Here's how the part is built. I have some questions about the finished solid (model axes, mm). A direction names the side the tool comes from. Coordinates: 2 decimals unless noted, no trailing zeros. Loops run counter-clockwise (first coordinate to the right, second up) from the corner with the lowest first, then second, coordinate; pieces in that order, holes last. Notation, with made-up numbers: (82.5, 0) - (120.5, 0) arc R24 cw to (120.5, 35) - close; hole circle Ø7 at (47, 30). An arc over 180 degrees is marked (long way). Use a Markdown table: item, result.
```python
from build123d import *

# Parameters (mm, degrees)
SKETCH2_R           = 3.429
BOSS_EXTRUDE1_DEPTH = 6.35
SKETCH6_R           = 3.429
BOSS_EXTRUDE2_DEPTH = 6.35
SKETCH7_R           = 2.63525
BOSS_EXTRUDE3_DEPTH = 11.43
CUT_EXTRUDE2_START  = -6.35
CUT_EXTRUDE2_DEPTH  = 6.35
FILLET2_R           = 2.54
FILLET3_R           = 0.508
SKETCH12_R          = 3.302
CUT_EXTRUDE3_DEPTH  = 15.875
SKETCH13_R          = 3.302
CUT_EXTRUDE4_DEPTH  = 15.875


with BuildPart() as part:
    # Sketch2 → Boss-Extrude1 (new body)
    with BuildSketch(Plane(origin=(0, 0, 0), x_dir=(1, 0, 0), z_dir=(0, 1, 0))):
        with BuildLine():
            Line((-7.239, 0), (-7.239, 10.16))
            ThreePointArc((-7.239, 10.16), (0, 17.399), (7.239, 10.16))
            Line((7.239, 10.16), (7.239, 0))
            Line((7.239, 0), (-7.239, 0))
        make_face()
        with Locations(Location((0, 10.16, 0), (0, 0, 270))):
            Circle(SKETCH2_R, mode=Mode.SUBTRACT)
    extrude(amount=BOSS_EXTRUDE1_DEPTH)



with BuildPart() as body_2:
    # Sketch6 → Boss-Extrude2 (new body)
    with BuildSketch(Plane(origin=(0, 31.242, 0), x_dir=(-1, 0, 0), z_dir=(0, -1, 0))):
        with BuildLine():
            Line((7.239, 0), (-7.239, 0))
            Line((-7.239, 0), (-7.239, 10.16))
            ThreePointArc((-7.239, 10.16), (0, 17.399), (7.239, 10.16))
            Line((7.239, 10.16), (7.239, 0))
        make_face()
        with Locations(Location((0, 10.16, 0), (0, 0, 270))):
            Circle(SKETCH6_R, mode=Mode.SUBTRACT)
    extrude(amount=BOSS_EXTRUDE2_DEPTH)


with BuildPart() as part_1:
    add(part.part)

    add(body_2.part)  # Boss-Extrude3 merges body 2
    # Sketch7 → Boss-Extrude3 (add)
    with BuildSketch(Plane.XY):
        with BuildLine():
            Line((11.43, -0.73025), (-8.89, -0.73025))
            ThreePointArc((-8.89, -0.73025), (-10.686051224, 0.013698776), (-11.43, 1.80975))
            Line((-11.43, 1.80975), (-11.43, 17.427370456))
            ThreePointArc((-11.43, 17.427370456), (-11.929359281, 18.939780934), (-13.231090909, 19.857517232))
            ThreePointArc((-13.231090909, 19.857517232), (-17.553942327, 26.691443265), (-11.43, 31.97225))
            Line((-11.43, 31.97225), (8.89, 31.97225))
            ThreePointArc((8.89, 31.97225), (10.686051224, 31.228301224), (11.43, 29.43225))
            Line((11.43, 29.43225), (11.43, 13.814629544))
            ThreePointArc((11.43, 13.814629544), (11.929359281, 12.302219066), (13.231090909, 11.384482768))
            ThreePointArc((13.231090909, 11.384482768), (17.553942327, 4.550556735), (11.43, -0.73025))
        make_face()
        with Locations((-11.43, 25.781)):
            Circle(SKETCH7_R, mode=Mode.SUBTRACT)
        with Locations(Location((11.43, 5.461, 0), (0, 0, 180))):
            Circle(SKETCH7_R, mode=Mode.SUBTRACT)
    extrude(amount=BOSS_EXTRUDE3_DEPTH)

    # Sketch11 → Cut-Extrude2 (cut)
    with BuildSketch(Plane.XY.offset(11.43).offset(CUT_EXTRUDE2_START)):
        with BuildLine():
            Line((11.43, 18.923), (-11.91702843, 18.923))
            ThreePointArc((-11.91702843, 18.923), (-11.554824252, 18.213834763), (-11.43, 17.427370456))
            Line((-11.43, 17.427370456), (-11.43, 12.065))
            Line((-11.43, 12.065), (12.128697076, 12.065))
            ThreePointArc((12.128697076, 12.065), (11.611132748, 12.872639477), (11.43, 13.814629544))
            Line((11.43, 13.814629544), (11.43, 18.923))
        make_face()
    extrude(amount=CUT_EXTRUDE2_DEPTH, mode=Mode.SUBTRACT)

    # Fillet2
    fillet2_edges = [part_1.edges().sort_by_distance(p)[0] for p in [
        (11.43, 18.923, 8.255),
        (-11.43, 12.065, 8.255),
    ]]
    fillet(fillet2_edges, radius=FILLET2_R)

    # Fillet3
    fillet3_edges = [part_1.edges().sort_by_distance(p)[0] for p in [
        (-10.686051224, 11.321051224, 5.08),
        (1.619348538, 12.065, 5.08),
    ]]
    fillet(fillet3_edges, radius=FILLET3_R)
    fillet3_2_edges = [part_1.edges().sort_by_distance(p)[0] for p in [
        (-1.513514215, 18.923, 5.08),
        (10.686051224, 19.666948776, 5.08),
    ]]
    fillet(fillet3_2_edges, radius=FILLET3_R)
    fillet3_3_edges = [part_1.edges().sort_by_distance(p)[0] for p in [
        (0, 0, 0),
    ]]
    fillet(fillet3_3_edges, radius=FILLET3_R)
    fillet3_4_edges = [part_1.edges().sort_by_distance(p)[0] for p in [
        (0, 6.35, 0),
    ]]
    fillet(fillet3_4_edges, radius=FILLET3_R)
    fillet3_5_edges = [part_1.edges().sort_by_distance(p)[0] for p in [
        (0, 31.242, 0),
    ]]
    fillet(fillet3_5_edges, radius=FILLET3_R)
    fillet3_6_edges = [part_1.edges().sort_by_distance(p)[0] for p in [
        (0, 24.892, 0),
    ]]
    fillet(fillet3_6_edges, radius=FILLET3_R)
    fillet3_7_edges = [part_1.edges().sort_by_distance(p)[0] for p in [
        (7.239, 28.067, 0),
    ]]
    fillet(fillet3_7_edges, radius=FILLET3_R)
    fillet3_8_edges = [part_1.edges().sort_by_distance(p)[0] for p in [
        (-7.239, 28.067, 0),
    ]]
    fillet(fillet3_8_edges, radius=FILLET3_R)
    fillet3_9_edges = [part_1.edges().sort_by_distance(p)[0] for p in [
        (7.239, 3.175, 0),
    ]]
    fillet(fillet3_9_edges, radius=FILLET3_R - 0.0001)  # a hair under: the kernel refuses the full size
    fillet3_10_edges = [part_1.edges().sort_by_distance(p)[0] for p in [
        (-7.239, 3.175, 0),
    ]]
    fillet(fillet3_10_edges, radius=FILLET3_R - 0.0001)  # a hair under: the kernel refuses the full size

    # Sketch12 → Cut-Extrude3 (cut)
    with BuildSketch(Plane(origin=(11.43, 0, 0), x_dir=(0, 0, -1), z_dir=(1, 0, 0))):
        with Locations((-5.715, 25.447625)):
            Circle(SKETCH12_R)
    extrude(amount=-CUT_EXTRUDE3_DEPTH, mode=Mode.SUBTRACT)

    # Sketch13 → Cut-Extrude4 (cut)
    with BuildSketch(Plane.ZY.offset(11.43)):
        with Locations((5.715, 5.667375)):
            Circle(SKETCH13_R)
    extrude(amount=-CUT_EXTRUDE4_DEPTH, mode=Mode.SUBTRACT)


solid = part_1.part
```
Q1. Which directions (+Z, -Z, +X, -X, +Y, -Y) give clear straight access to the entire face, cutting with the end or side of a thin tool? Please do faces 1 (the face through (7.239, 28, -5)), 2 (the face through (0, 6.35, -5)), 3 (the face through (-10.706, 11.301, 8.55)), 4 (the face through (0, 0, -5)).
Check values:
| item | result |
|---|---|
| face 1 | -Z, +X, +Y, -Y |
| face 2 | -Z, +X, -X |
| face 3 | +Z, -X |
| face 4 | -Z, +X, -X, -Y |
Q2. Will these pins go through, and if not, where does the flat tip stop? P1, Ø3, axis at x = -0.5, z = -4.5, coming from the -Y side; P2, Ø9, axis at x = 0, z = -10.16, coming from the +Y side; P3, Ø7.5, axis at y = 25.45, z = 5.72, coming from the -X side; P4, Ø2, axis at x = -1.5, y = 21, coming from the -Z side.
Check values:
| item | result |
|---|---|
| P1 | y = 0 |
| P2 | y = 31.24 |
| P3 | x = -17.62 |
| P4 | z = 0 |
Q3. I want a section at A-A, the plane z = -4.5. Write out the boundary of the cut face in (x, y).
Check values:
| item | result |
|---|---|
| outline | (-7.24, 0) - (7.24, 0) - (7.24, 6.35) - (-7.24, 6.35) - close; (-7.24, 24.89) - (7.24, 24.89) - (7.24, 31.24) - (-7.24, 31.24) - close |
Q4. Please list where these lines run through material, in increasing order: L1, parallel to Y at x = 5, z = -13.5; L2, parallel to X at y = 27.25, z = -10.16; L3, parallel to Y at x = 6.5, z = 8 (3 decimals). Write a range as from..to.
Check values:
| item | result |
|---|---|
| L1 | 0..6.35, 24.89..31.24 |
| L2 | -7.24..-3.43, 3.43..7.24 |
| L3 | -0.73..12.065, 18.923..23.064, 27.831..31.972 |
Q5. I want a section at D-D, the plane z = -7.5. Write out the boundary of the cut face in (x, y).
Check values:
| item | result |
|---|---|
| outline | (-7.24, 0) - (-2.16, 0) - (-2.16, 6.35) - (-7.24, 6.35) - close; (-7.24, 24.89) - (-2.16, 24.89) - (-2.16, 31.24) - (-7.24, 31.24) - close; (2.16, 0) - (7.24, 0) - (7.24, 6.35) - (2.16, 6.35) - close; (2.16, 24.89) - (7.24, 24.89) - (7.24, 31.24) - (2.16, 31.24) - close |
Q6. If we mould it in two halves opening along Y, with no side actions, what happens to faces 5 (the face through (3, 6, 11.43)), 6 (the face through (-3.604, 4.403, 8.765)), 7 (the face through (12.148, 12.045, 4.365))? For each: pulls with the +Y half, pulls with the -Y half, needs draft (parallel to the pull), parting line crosses it, or undercut.
Check values:
| item | result |
|---|---|
| face 5 | needs draft |
| face 6 | undercut |
| face 7 | pulls with the +Y half |
Q7. I want a section at C-C, the plane z = 8.5. Write out the boundary of the cut face in (x, y) (1 decimal).
Check values:
| item | result |
|---|---|
| outline | (-13.2, 19.9) arc R2.5 cw to (-11.9, 18.9) - (8.9, 18.9) arc R2.5 ccw to (11.4, 21.5) - (11.4, 23.7) - (-4.4, 23.7) - (-4.4, 27.2) - (11.4, 27.2) - (11.4, 29.4) arc R2.5 ccw to (8.9, 32) - (-11.4, 32) arc R6.2 ccw to start; (-11.4, 1.8) arc R2.5 ccw to (-8.9, -0.7) - (11.4, -0.7) arc R6.2 ccw to (13.2, 11.4) arc R2.5 cw to (12.1, 12.1) - (-8.9, 12.1) arc R2.5 ccw to (-11.4, 9.5) - (-11.4, 7.4) - (4.4, 7.4) - (4.4, 3.9) - (-11.4, 3.9) - close; hole circle Ø5.3 at (-11.4, 25.8); hole circle Ø5.3 at (11.4, 5.5) |
Q8. I want a section at B-B, the plane x = -1. Give the number of separate pieces and of enclosed holes in the cut face, then the cut area to 3 significant figures.
Check values:
| item | result |
|---|---|
| separate pieces | 3 |
| enclosed holes | 2 |
| area | 399 mm^2 |
